```python
from build123d import *

# Parameters (mm, degrees)
SKETCH1_R            = 38.1
SKETCH1_R_2          = 27.727172307
BOSS_EXTRUDE1_DEPTH  = 26.9875
BOSS_EXTRUDE2_START  = 5.5118
SKETCH2_R            = 38.1
SKETCH2_R_2          = 22.0345
BOSS_EXTRUDE2_DEPTH  = 5.5118
SKETCH3_R            = 38.1
SKETCH3_R_2          = 22.0345
BOSS_EXTRUDE3_DEPTH  = 26.9875
BOSS_EXTRUDE4_DEPTH  = 2.3876
BOSS_EXTRUDE5_START  = 2.2098
SKETCH5_R            = 38.1
SKETCH5_R_2          = 17.526
BOSS_EXTRUDE5_DEPTH  = 2.2098
SKETCH7_R            = 24.60625
CUT_EXTRUDE1_DEPTH   = 1.778
SKETCH8_R            = 38.1
SKETCH8_R_2          = 6.5151
BOSS_EXTRUDE6_DEPTH  = 5.969
SKETCH9_R            = 38.1
SKETCH9_R_2          = 5.0165
BOSS_EXTRUDE7_DEPTH  = 5.2578
SKETCH10_R           = 38.1
BOSS_EXTRUDE8_DEPTH  = 1.5875
BOSS_EXTRUDE9_REACH  = 74.802
SKETCH12_R           = 41.275
SKETCH12_R_2         = 31.75
BOSS_EXTRUDE10_DEPTH = 12.319


with BuildPart() as part:
    # Sketch1 → Boss-Extrude1 (new body)
    with BuildSketch(Plane(origin=(0, 0, 0), x_dir=(0, 0, -1), z_dir=(1, 0, 0))):
        Circle(SKETCH1_R)
        Circle(SKETCH1_R_2, mode=Mode.SUBTRACT)
    extrude(amount=BOSS_EXTRUDE1_DEPTH)

    # Sketch2 → Boss-Extrude2 (add)
    with BuildSketch(Plane.ZY.offset(BOSS_EXTRUDE2_START)):
        Circle(SKETCH2_R)
        Circle(SKETCH2_R_2, mode=Mode.SUBTRACT)
    extrude(amount=-BOSS_EXTRUDE2_DEPTH)

    # Sketch3 → Boss-Extrude3 (add)
    with BuildSketch(Plane(origin=(26.9875, 0, 0), x_dir=(0, 0, -1), z_dir=(1, 0, 0))):
        with Locations(Location((0, 0, 0), (0, 0, 180))):
            Circle(SKETCH3_R)
        with Locations(Location((0, 0, 0), (0, 0, 180))):
            Circle(SKETCH3_R_2, mode=Mode.SUBTRACT)
    extrude(amount=BOSS_EXTRUDE3_DEPTH)

    # Sketch4 → Boss-Extrude4 (add)
    with BuildSketch(Plane(origin=(0, 0, 0), x_dir=(0, 0, -1), z_dir=(1, 0, 0))):
        with BuildLine():
            Line((-2.1336, 21.930958513), (-2.1336, 27.727172307))
            Line((-2.1336, 27.727172307), (2.1336, 27.727172307))
            Line((2.1336, 27.727172307), (2.1336, 21.930958513))
            ThreePointArc((2.1336, 21.930958513), (0, 22.0345), (-2.1336, 21.930958513))
        make_face()
    boss_extrude4 = extrude(amount=BOSS_EXTRUDE4_DEPTH)

    # Mirror1: Boss-Extrude4 across plane
    add(boss_extrude4.mirror(Plane.ZX))

    # Sketch5 → Boss-Extrude5 (add)
    with BuildSketch(Plane.ZY.offset(5.5118).offset(BOSS_EXTRUDE5_START)):
        Circle(SKETCH5_R)
        Circle(SKETCH5_R_2, mode=Mode.SUBTRACT)
    extrude(amount=-BOSS_EXTRUDE5_DEPTH)

    # Sketch7 → Cut-Extrude1 (cut)
    with BuildSketch(Plane.ZY.offset(-39.4589)):
        Circle(SKETCH7_R)
    extrude(amount=-CUT_EXTRUDE1_DEPTH, mode=Mode.SUBTRACT)

    # Sketch8 → Boss-Extrude6 (add)
    with BuildSketch(Plane(origin=(53.975, 0, 0), x_dir=(0, 0, -1), z_dir=(1, 0, 0))):
        with Locations(Location((0, 0, 0), (0, 0, 180))):
            Circle(SKETCH8_R)
        Circle(SKETCH8_R_2, mode=Mode.SUBTRACT)
    extrude(amount=BOSS_EXTRUDE6_DEPTH)

    # Sketch9 → Boss-Extrude7 (add)
    with BuildSketch(Plane(origin=(59.944, 0, 0), x_dir=(0, 0, -1), z_dir=(1, 0, 0))):
        with Locations(Location((0, 0, 0), (0, 0, 180))):
            Circle(SKETCH9_R)
        Circle(SKETCH9_R_2, mode=Mode.SUBTRACT)
    extrude(amount=BOSS_EXTRUDE7_DEPTH)

    # Sketch10 → Boss-Extrude8 (add)
    with BuildSketch(Plane(origin=(65.2018, 0, 0), x_dir=(0, 0, -1), z_dir=(1, 0, 0))):
        with Locations(Location((0, 0, 0), (0, 0, 180))):
            Circle(SKETCH10_R)
    extrude(amount=BOSS_EXTRUDE8_DEPTH)

    # Sketch11 → Boss-Extrude9 (add, up to next)
    with BuildSketch(Plane.ZY.offset(-41.2369), mode=Mode.PRIVATE) as boss_extrude9_sk1:
        with BuildLine():
            Line((1.8034, -21.960576921), (1.8034, -24.60625))
            Line((1.8034, -24.60625), (-1.8034, -24.60625))
            Line((-1.8034, -24.60625), (-1.8034, -21.960576921))
            ThreePointArc((-1.8034, -21.960576921), (0, -22.0345), (1.8034, -21.960576921))
        make_face()
    boss_extrude9_tool1 = extrude(boss_extrude9_sk1.sketch, amount=BOSS_EXTRUDE9_REACH, mode=Mode.PRIVATE) - part.part
    boss_extrude9 = boss_extrude9_tool1.solids().sort_by_distance((41.2369, -23.307969, 0))[0]
    add(boss_extrude9)

    # Mirror2: Boss-Extrude9 across plane
    add(boss_extrude9.mirror(Plane.ZX))

    # Sketch12 → Boss-Extrude10 (add)
    with BuildSketch(Plane.ZY.offset(7.7216)):
        with Locations(Location((0, 0, 0), (0, 0, 180))):
            Circle(SKETCH12_R)
        with Locations(Location((0, 0, 0), (0, 0, 180))):
            Circle(SKETCH12_R_2, mode=Mode.SUBTRACT)
    extrude(amount=BOSS_EXTRUDE10_DEPTH)


solid = part.part
```
Part model, mm, in its own coordinate system. A direction names the side the tool comes from. Round coordinates to 2 decimals unless told otherwise and drop trailing zeros. Loops run counter-clockwise (first coordinate to the right, second up) from the corner with the lowest first, then second, coordinate; pieces in that order, holes last. Notation, with made-up numbers: (84, 39.5) -> (99, 39.5) arc R27 cw to (99, 73.5) -> close; hole circle Ø3 at (39, 42.5). An arc over 180 degrees is marked (long way). Use CSV: the item, a comma, the result in double quotes. Start each with the question number.
1) Cut at A-A, the plane x = 9. Write the cut outline in (y, z), plus the area to 3 significant figures.
2) Drop flat-ended pins along their axis: P1, Ø6.5, axis at y = 0.5, z = 1, coming from the -X side; P2, Ø1, axis at x = 13, z = -9.5, coming from the -Y side; P3, Ø12, axis at x = 5.5, y = -19.5, coming from the +Z side. Give the stop position or say it passes through.
3) Cut at C-C, the plane y = -33. Write the cut outline in (x, z).
4) Pull direction Y, two halves, no side cores. Call faces 4 (the cylindrical face through (-13.795, -40.924, 5.373)), 5 (the flat face through (66.789, -1, -1)), 6 (the flat face through (59.944, 5, 2)): +Y half, -Y half, draft (parallel to the pull), parting line (faces both ways), or undercut.
5) Which spindle directions (+Z, -Z, +X, -X, +Y, -Y) get a long thin tool onto all of the face, cutting with end or side? Do faces 1 (the flat face through (1, -25, 2.134)), 2 (the cylindrical face through (-13.795, 30.995, 6.883)), 3 (the flat face through (-7.722, 36.5, -12)). Say none if no direction does.
6) Wall check: L1, parallel to X at y = -7, z = -23.5; L2, parallel to Y at x = 21, z = 0; L3, parallel to Y at x = 33, z = 0. Give the ranges that are in metal, low to high. Write a range as [from, to].
7) Cut at D-D, the plane x = 46.5. Write the cut outline in (y, z).
Determined:
1,outline,"circle Ø76.2 at (0, 0); hole circle Ø55.45 at (0, 0)"
1,area,"2,150 mm2"
2,P1,"stops at x = 65.2"
2,P2,"stops at y = -37.02"
2,P3,"stops at z = 35.63"
3,outline,"(-20.04, -24.79) -> (-7.72, -24.79) -> (-7.72, -19.04) -> (66.79, -19.04) -> (66.79, 19.04) -> (-7.72, 19.04) -> (-7.72, 24.79) -> (-20.04, 24.79) -> close"
4,face 4,"parting line"
4,face 5,"draft"
4,face 6,"undercut"
5,face 1,"none"
5,face 2,"-X"
5,face 3,"+X"
6,L1,"x = [-7.72, 0], [26.99, 39.46], [41.24, 66.79]"
6,L2,"y = [-38.1, -27.73], [27.73, 38.1]"
6,L3,"y = [-38.1, -22.03], [22.03, 38.1]"
7,outline,"circle Ø76.2 at (0, 0); hole circle Ø44.07 at (0, 0)"
